from build123d import *

# Parameters (mm, degrees)
F1_DEPTH = 12.3
F2_W     = 8
F2_H     = 2
F2_W_2   = 5
F3_DEPTH = 9.951001
F5_DEPTH = 10.901


with BuildPart() as f1:
    # F0 (on Front) → F1 (new body)
    with BuildSketch(Plane.XZ):
        Polygon((4.5, 8.4), (0, 8.4), (0, 0), (18.9, 0), (18.9, 6.7), (10.149998, 9.950001), align=None)
    extrude(amount=F1_DEPTH)

    # F2 (on face) → F3 (cut, through all)
    with BuildSketch(Plane(origin=(0, 0, 0), x_dir=(1, 0, 0), z_dir=(0, 0, -1))):
        with Locations((4, 6.15)):
            Rectangle(F2_W, F2_H)
        with Locations((16.4, 6.15)):
            Rectangle(F2_W_2, F2_H)
    extrude(amount=-F3_DEPTH, mode=Mode.SUBTRACT)

    # F4 (on face) → F5 (cut, through all)
    with BuildSketch(Plane(origin=(8, 0, 0), x_dir=(0, -1, 0), z_dir=(-1, 0, 0))):
        with BuildLine():
            ThreePointArc((5.15, 4.2), (6.15, 3.2), (7.15, 4.2))
            ThreePointArc((7.15, 4.2), (6.15, 5.2), (5.15, 4.2))
        make_face()
    extrude(amount=-F5_DEPTH, mode=Mode.SUBTRACT)


solid = f1.part
Design review of the part built by this model. Coordinates are the model's own, in mm. A direction names the side the tool comes from. Coordinates: 2 decimals unless noted, no trailing zeros. Loops run counter-clockwise (first coordinate to the right, second up) from the corner with the lowest first, then second, coordinate; pieces in that order, holes last. Notation, with made-up numbers: M -4.5,10.5 L 41.5,10.5 A29 cw 41.5,49.5 Z; hole C 89.25,84.25 d4. An arc over 180 degrees is marked long. Answer as CSV lines item,"result".
Item 1: The part is to be moulded in two halves that separate along Y. For faces 1 (the face through (2, -3, 8.4)), 2 (the face through (9, 0, 4)), 3 (the face through (4, -7.15, 5)), say which applies: pulls with the +Y half, pulls with the -Y half, needs draft (parallel to the pull), parting line crosses it, or undercut.
Answer list:
face 1,"needs draft"
face 2,"pulls with the +Y half"
face 3,"undercut"
Item 2: Machinability: for faces 4 (the face through (8, -6, 2)), 5 (the face through (13.9, -6, 7)), 6 (the face through (18.9, -10, 3)), 7 (the face through (2, -10, 8.4)), which of the approach directions +Z, -Z, +X, -X, +Y, -Y give a long, thin tool a straight path to every point of the face, cutting with its end or side? Answer none if there is none.
Answer list:
face 4,"+Z, -Z, -X"
face 5,"+Z, -Z, +X"
face 6,"+Z, -Z, +X, +Y, -Y"
face 7,"+Z, -X, +Y, -Y"
Item 3: For P1, Ø6, axis at x = 14.5, y = -9.5, coming from the +Z side; P2, Ø2, axis at y = -9, z = 2.5, coming from the -X side; P3, Ø1.3, axis at x = 2.5, y = -9, coming from the +Z side; P4, Ø1, axis at y = -6, z = 1.5, coming from the +X side, all flat-tipped, find the tip position at first contact; note any pin that passes through.
Answer list:
P1,"z = 9.45"
P2,"x = 0"
P3,"z = 8.4"
P4,"x = 13.9"
Item 4: Add section C-C on z = 3.75. State the section outline as (x, y) points.
Answer list:
outline,"M 0,-12.3 L 18.9,-12.3 L 18.9,-7.15 L 13.9,-7.15 L 13.9,-7.04 L 8,-7.04 L 8,-7.15 L 0,-7.15 Z; M 0,-5.15 L 8,-5.15 L 8,-5.26 L 13.9,-5.26 L 13.9,-5.15 L 18.9,-5.15 L 18.9,0 L 0,0 Z"
Item 5: Add section B-B on x = 3. State the section outline as (y, z) points.
Answer list:
outline,"M -12.3,0 L -7.15,0 L -7.15,8.4 L -12.3,8.4 Z; M -5.15,0 L 0,0 L 0,8.4 L -5.15,8.4 Z"
Item 6: Add section D-D on y = -3.25. State the section outline as (x, z) points.
Answer list:
outline,"M 0,0 L 18.9,0 L 18.9,6.7 L 10.15,9.95 L 4.5,8.4 L 0,8.4 Z"
Item 7: Add section A-A on y = -6.15. State the section outline as (x, z) points, plus the area to 3 significant figures.
Answer list:
outline,"M 8,0 L 13.9,0 L 13.9,3.2 L 8,3.2 Z; M 8,5.2 L 13.9,5.2 L 13.9,8.56 L 10.15,9.95 L 8,9.36 Z"
area,"43.7 mm²"
Item 8: For probe 1 along Y at (x, z) = (12.2, 4.2); probe 2 along Z at (x, y) = (11.75, -12), list the stretches that pass through material, from the lowest coordinate up.
Answer list:
probe 1,"-12.3 to -7.15, -5.15 to 0"
probe 2,"0 to 9.36"
